```python
from build123d import *

# Parameters (mm, degrees)
F1_DEPTH = 39
F2_R     = 2.5
F3_DEPTH = 2.748387
F4_W     = 10
F4_H     = 10
F5_DEPTH = 3


with BuildPart() as f1:
    # F0 (on Front) → F1 (new body, symmetric)
    with BuildSketch(Plane.XZ):
        Polygon((33.024074, -6.624926), (-2.974825, -6.624926), (-2.974825, -9.624926), (36.025175, -9.624926), (36.025175, 18.375074), (48.024074, 18.375074), (48.024074, 21.123461), (33.024074, 21.123461), align=None)
        Polygon((-2.974825, -9.624926), (-2.974825, -6.624926), (-38.973723, -6.624926), (-38.973723, 21.123461), (-53.973723, 21.123461), (-53.973723, 18.375074), (-41.974825, 18.375074), (-41.974825, -9.624926), align=None)
    extrude(amount=F1_DEPTH, both=True)

    # F2 (on face) → F3 (cut, through all)
    with BuildSketch(Plane.XY.offset(21.123461)):
        with Locations((42.024624, -24)):
            Circle(F2_R)
        with Locations((42.024624, 24)):
            Circle(F2_R)
        with Locations((-47.974274, 24)):
            Circle(F2_R)
        with Locations((-47.974274, -24)):
            Circle(F2_R)
    extrude(amount=-F3_DEPTH, mode=Mode.SUBTRACT)

    # F4 (on face) → F5 (cut, through all)
    with BuildSketch(Plane(origin=(0, 0, -9.624926), x_dir=(1, 0, 0), z_dir=(0, 0, -1))):
        with Locations((-31.473723, 31.5)):
            Rectangle(F4_W, F4_H)
        with Locations((-17.473723, 31.5)):
            Rectangle(F4_W, F4_H)
        with Locations((-3.473723, 31.5)):
            Rectangle(F4_W, F4_H)
        with Locations((10.526277, 31.5)):
            Rectangle(F4_W, F4_H)
        with Locations((24.526277, 31.5)):
            Rectangle(F4_W, F4_H)
        with Locations((10.526277, 18.965352)):
            Rectangle(F4_W, F4_H)
        with Locations((24.526277, 18.965352)):
            Rectangle(F4_W, F4_H)
        with Locations((-31.473723, 18.965352)):
            Rectangle(F4_W, F4_H)
        with Locations((-17.473723, 18.965352)):
            Rectangle(F4_W, F4_H)
        with Locations((-3.473723, 18.965352)):
            Rectangle(F4_W, F4_H)
        with Locations((10.526277, 6.430703)):
            Rectangle(F4_W, F4_H)
        with Locations((24.526277, 6.430703)):
            Rectangle(F4_W, F4_H)
        with Locations((-31.473723, 6.430703)):
            Rectangle(F4_W, F4_H)
        with Locations((-17.473723, 6.430703)):
            Rectangle(F4_W, F4_H)
        with Locations((-3.473723, 6.430703)):
            Rectangle(F4_W, F4_H)
        with Locations((10.526277, -6.103945)):
            Rectangle(F4_W, F4_H)
        with Locations((24.526277, -6.103945)):
            Rectangle(F4_W, F4_H)
        with Locations((-31.473723, -6.103945)):
            Rectangle(F4_W, F4_H)
        with Locations((-17.473723, -6.103945)):
            Rectangle(F4_W, F4_H)
        with Locations((-3.473723, -6.103945)):
            Rectangle(F4_W, F4_H)
        with Locations((10.526277, -18.638594)):
            Rectangle(F4_W, F4_H)
        with Locations((24.526277, -18.638594)):
            Rectangle(F4_W, F4_H)
        with Locations((-31.473723, -18.638594)):
            Rectangle(F4_W, F4_H)
        with Locations((-17.473723, -18.638594)):
            Rectangle(F4_W, F4_H)
        with Locations((-3.473723, -18.638594)):
            Rectangle(F4_W, F4_H)
        with Locations((10.526277, -31.173242)):
            Rectangle(F4_W, F4_H)
        with Locations((24.526277, -31.173242)):
            Rectangle(F4_W, F4_H)
        with Locations((-31.473723, -31.173242)):
            Rectangle(F4_W, F4_H)
        with Locations((-17.473723, -31.173242)):
            Rectangle(F4_W, F4_H)
        with Locations((-3.473723, -31.173242)):
            Rectangle(F4_W, F4_H)
    extrude(amount=-F5_DEPTH, mode=Mode.SUBTRACT)


solid = f1.part
```
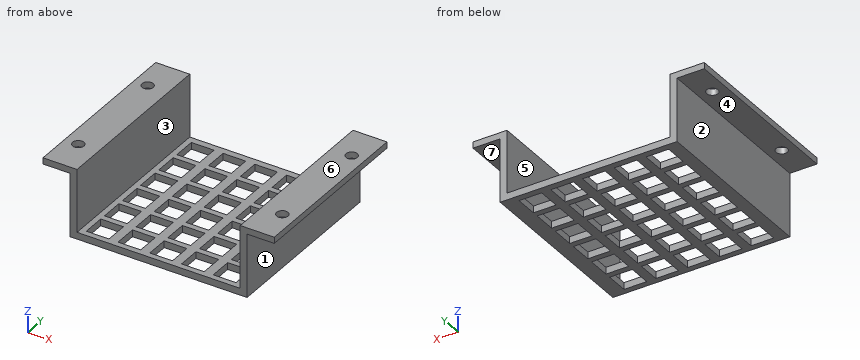
Input: part model. Units: mm. Frame: model coordinates. Face numbers are marked on the shaded views. A direction names the side the tool comes from. Give positions to 0.01 mm unless a question says otherwise; leave off trailing zeros. Loops run counter-clockwise (first coordinate to the right, second up) from the corner with the lowest first, then second, coordinate; pieces in that order, holes last.
1) Reachability of the marked faces 5, 6 and 7 from +Z, -Z, +X, -X, +Y, -Y: full face, straight path, thin tool, end or side. Return the list, or none.
A:
face 5: +Z, +Y, -Y
face 6: +Z, +X, -X, +Y, -Y
face 7: -Z, +X, +Y, -Y
2) Section query A-A on x = 24. Return the cut outline in (y, z).
A:
outline: (-39, -9.62) - (-36.5, -9.62) - (-36.5, -6.62) - (-39, -6.62) - close; (-26.5, -9.62) - (-23.97, -9.62) - (-23.97, -6.62) - (-26.5, -6.62) - close; (-13.97, -9.62) - (-11.43, -9.62) - (-11.43, -6.62) - (-13.97, -6.62) - close; (-1.43, -9.62) - (1.1, -9.62) - (1.1, -6.62) - (-1.43, -6.62) - close; (11.1, -9.62) - (13.64, -9.62) - (13.64, -6.62) - (11.1, -6.62) - close; (23.64, -9.62) - (26.17, -9.62) - (26.17, -6.62) - (23.64, -6.62) - close; (36.17, -9.62) - (39, -9.62) - (39, -6.62) - (36.17, -6.62) - close
3) Section query C-C on y = -32. Count the separate pieces of the cut face and the enclosed holes in it, and give its area (3 significant figures).
A:
separate pieces: 6
enclosed holes: 0
area: 317 mm2
4) Contact query for flat-ended pins moving along their axis: pin 1 (0.9 mm diameter, centred on y = -5.5, z = -8, fed in from +X); pin 2 (1.5 mm diameter, centred on y = -5, z = -9, fed in from -X); pin 3 (8 mm diameter, centred on x = -19, y = -28, fed in from +Z). Output: stop coordinate, or through.
A:
pin 1: stops at x = 36.03
pin 2: stops at x = -41.97
pin 3: stops at z = -6.62
5) Section query B-B on z = 8. Return the cut outline in (x, y), and give its area (3 significant figures).
A:
outline: (-41.97, -39) - (-38.97, -39) - (-38.97, 39) - (-41.97, 39) - close; (33.02, -39) - (36.03, -39) - (36.03, 39) - (33.02, 39) - close
area: 468 mm2
6) Line query: L1, parallel to X at y = 6.5, z = -8; L2, parallel to X at y = -23, z = 11; L3, parallel to X at y = -8, z = 18.5. Output: solid intervals per line, ascending.
A:
L1: x = -41.97 to -36.47, -26.47 to -22.47, -12.47 to -8.47, 1.53 to 5.53, 15.53 to 19.53, 29.53 to 36.03
L2: x = -41.97 to -38.97, 33.02 to 36.03
L3: x = -53.97 to -38.97, 33.02 to 48.02
7) Mould query, pull axis X, two halves, no side actions, for the marked faces 1, 2, 3 and 4. Classes: released by +X, released by -X, zero draft, split by the parting line, or undercut.
A:
face 1: released by +X
face 2: released by -X
face 3: undercut
face 4: zero draft
